Autodesk Fusion 360 part; units mm, degrees
sketch "Sketch1" plane through (0, 0, 0) normal (0, 0, 1) x (1, 0, 0)
  circle A0 centre (0, 0) radius 27.5
  dimension "d1" = 55
extrude "Extrude1" add sketch "Sketch1" along normal blind 40
sketch "Sketch2" plane through (0, 0, 40) normal (0, 0, 1) x (-1, 0, 0)
  circle A0 centre (0, 0) radius 27.5
  line L0 (0, -27.5) -> (-31, -27.5)
  line L1 (-31, -27.5) -> (-31, 40.6198)
  line L2 (0, 27.5) -> (-33.618, 27.5)
  line L3 (0, -27.5) -> (31, -27.5)
  line L4 (31, -27.5) -> (31, 43)
  line L5 (0, 27.5) -> (37, 27.5)
  dimension "d4" = 90
  dimension "d5" = 31
extrude "Extrude2" add sketch "Sketch2" along normal blind 70
sketch "Sketch3" plane through (0, 0, 110) normal (0, 0, 1) x (-1, 0, 0)
  line L0 (-31, -27.5) -> (31, -27.5)
  line L1 (31, -27.5) -> (31, 27.5)
  line L2 (31, 27.5) -> (-31, 27.5)
  line L3 (-31, 27.5) -> (-31, -27.5)
  circle A0 centre (0, 0) radius 5
  dimension "d8" = 10
extrude "Extrude3" add sketch "Sketch3" along normal blind 80 contours A0
sketch "Sketch4" plane through (0, 0, 0) normal (0, 1, 0) x (1, 0, 0)
chamfer "Chamfer1" distance 1 angle 45 1 edges at (4.6616, 1.8081, 190)
fillet "Fillet1" radius 5 4 edges at (31, -27.5, 75) (31, 27.5, 75) (-31, 27.5, 75) (-31, -27.5, 75)
The listing builds one solid part. Answer for the finished solid, in the listing's coordinates (mm). A direction names the side the tool comes from. Give positions to 0.01 mm unless a question says otherwise; leave off trailing zeros. Loops run counter-clockwise (first coordinate to the right, second up) from the corner with the lowest first, then second, coordinate; pieces in that order, holes last. Notation, with made-up numbers: (-2.5, 3) - (56.5, 3) arc R20 ccw to (56.5, 19) - close; hole circle Ø7 at (-19.75, 7). An arc over 180 degrees is marked (long way). Use one line per item in the form item = value.
1. Find the intervals of material crossed by line 1 along Z through (x, y) = (12.5, -19.5); line 2 along X through (y, z) = (3, 155); line 3 along Z through (x, y) = (17, -22), in increasing order. Write a range as [from, to].
Calculated:
line_1 = [0, 110]
line_2 = [-4, 4]
line_3 = [40, 110]
2. Given pin 1 Ø8 at (y, z) = (6.5, 24) entering from -X; pin 2 Ø1 at (y, z) = (11, 36) entering from -X; pin 3 Ø16.5 at (x, y) = (-14, -9) entering from +Z, each flat-ended and moving along its own axis, determine where each tip first touches the part or whether it passes through.
Calculated:
pin_1 = -27.39
pin_2 = -25.42
pin_3 = 110
3. Section B-B on y = 0 is taken. Give the vertices of the cut face in (x, z), then the cut area to 3 significant figures.
Calculated:
outline = (-31, 40) - (-27.5, 40) - (-27.5, 0) - (27.5, 0) - (27.5, 40) - (31, 40) - (31, 110) - (5, 110) - (5, 189) - (4, 190) - (-4, 190) - (-5, 189) - (-5, 110) - (-31, 110) - close
area = 7,340 mm^2
4. Which of the six approach directions +Z, -Z, +X, -X, +Y, -Y give full straight-line access (tool end or side, diameter ignored) to faces 1 (the face through (1.08, -4.88, 148.95)), 2 (the face through (-28, 0, 40)), 3 (the face through (28, 0, 40))?
Calculated:
face_1 = +Z
face_2 = -Z, -X
face_3 = -Z, +X
5. Section D-D on y = 9.5 is taken. Give the vertices of the cut face in (x, z).
Calculated:
outline = (-31, 40) - (-25.81, 40) - (-25.81, 0) - (25.81, 0) - (25.81, 40) - (31, 40) - (31, 110) - (-31, 110) - close
6. Section C-C on z = 172 is taken. Give the vertices of the cut face in (x, y).
Calculated:
outline = circle Ø10 at (0, 0)
7. Section A-A on x = 18.5 is taken. Give the vertices of the cut face in (y, z), then the cut area to 3 significant figures.
Calculated:
outline = (-27.5, 40) - (-20.35, 40) - (-20.35, 0) - (20.35, 0) - (20.35, 40) - (27.5, 40) - (27.5, 110) - (-27.5, 110) - close
area = 5,480 mm^2
